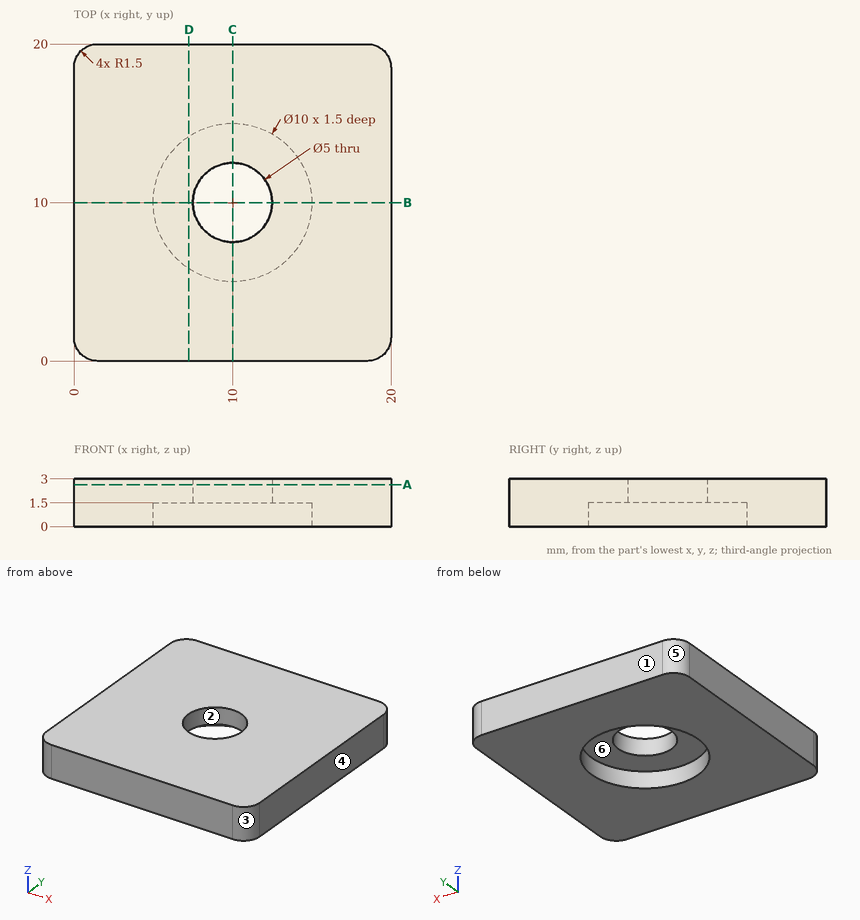
For this review, use the dimensioned drawing (mm, ordinates from the lowest corner) and the shaded views. A direction names the side the tool comes from. Give positions to 0.01 mm unless a question says otherwise; leave off trailing zeros. Order: outer loops, then holes, each group sorted by start corner. A loop starts at its lowest first (then second) coordinate and runs counter-clockwise, first axis right, second up. Notation, with made-up numbers: M -21.75,78 L 27.25,78 A20 ccw 27.25,114 Z; hole C 9.25,20 d1. An arc over 180 degrees is marked long. One line per question, with ' | ' between items. Start each with the question number.
1) Consider section A-A, the plane z = 2.65. Give the boundary of the cut face in (x, y), then the cut area to 3 significant figures.
2) Wall thickness on L1, parallel to Y at x = 10, z = 2.6; L2, parallel to Z at x = 11.75, y = 6.5: over which ranges is each line inside the solid? List them lowest first. Write a range as from..to.
3) Consider section D-D, the plane x = 7.25. Give the boundary of the cut face in (y, z).
4) For the marked faces 5 and 6, list the 3-axis set-ups (+Z, -Z, +X, -X, +Y, -Y) from which the entire face can be reached by the end or side of a thin tool; tool diameter is ignored.
5) Clearance check with a flat-ended pin moving along its axis: P1, Ø5, axis at x = 11, y = 10, coming from the -Z side. State where the tip first meets the part, or that it passes through.
6) Consider section B-B, the plane y = 10. Give the boundary of the cut face in (x, z).
7) Mouldability with a two-part tool opening along Y and no side actions: class the marked faces 1, 2, 3 and 4 as pulls with the +Y half, pulls with the -Y half, needs draft (parallel to the pull), parting line crosses it, or undercut.
Found:
1) outline: M 0,1.5 A1.5 ccw 1.5,0 L 18.5,0 A1.5 ccw 20,1.5 L 20,18.5 A1.5 ccw 18.5,20 L 1.5,20 A1.5 ccw 0,18.5 Z; hole C 10,10 d5 | area: 378 mm²
2) L1: y = 0..7.5, 12.5..20 | L2: z = 1.5..3
3) outline: M 0,0 L 5.82,0 L 5.82,1.5 L 14.18,1.5 L 14.18,0 L 20,0 L 20,3 L 0,3 Z
4) face 5: +Z, -Z, -X, +Y | face 6: -Z
5) P1: stops at z = 1.5
6) outline: M 0,0 L 5,0 L 5,1.5 L 7.5,1.5 L 7.5,3 L 0,3 Z; M 12.5,1.5 L 15,1.5 L 15,0 L 20,0 L 20,3 L 12.5,3 Z
7) face 1: pulls with the +Y half | face 2: undercut | face 3: pulls with the -Y half | face 4: needs draft
